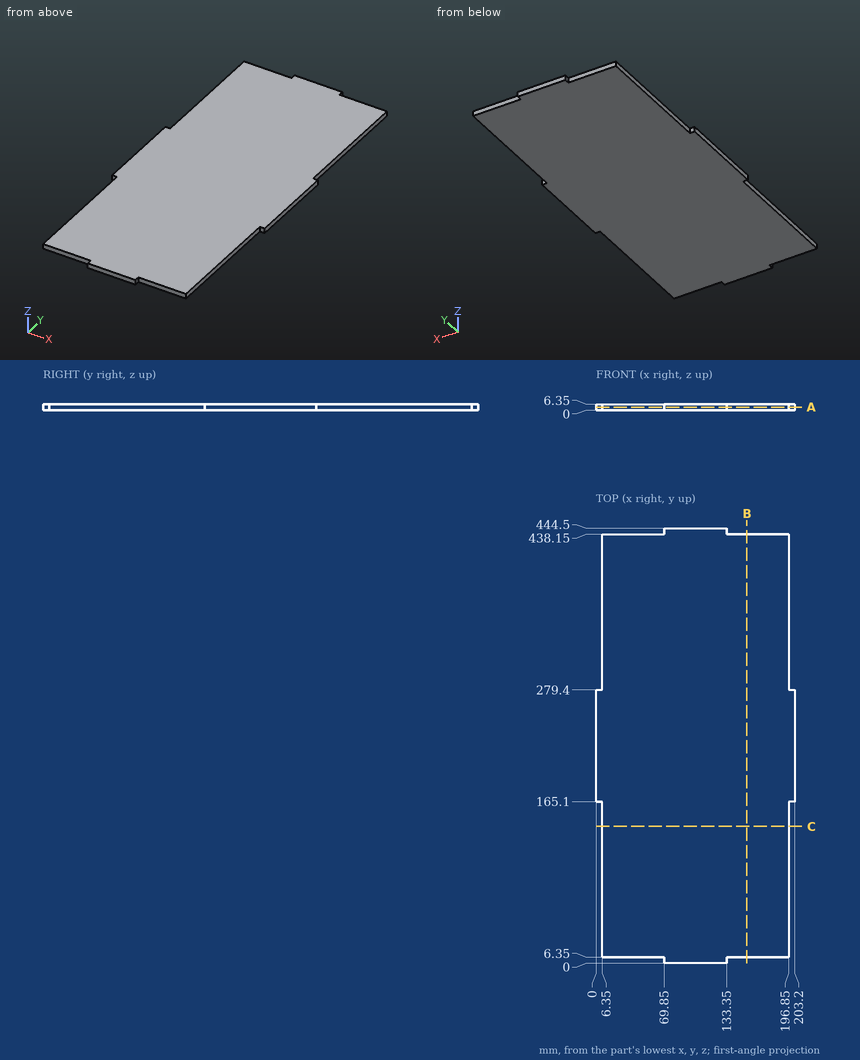
Could you check a few things on this drawing? It's one solid part, dimensions in mm from its lowest x, y, z. Give positions to 0.01 mm unless a question says otherwise; leave off trailing zeros. Order: outer loops, then holes, each group sorted by start corner. A loop starts at its lowest first (then second) coordinate and runs counter-clockwise, first axis right, second up. Notation, with made-up numbers: M -31,71.25 L 3,71.25 A32 cw 3,98.25 Z; hole C -15,-20.5 d11. An arc over 180 degrees is marked long. Use one line per item in the form item = value.
Item 1: If I drill on line 1 along X through (y, z) = (107.5, 0.5); line 2 along Y through (x, z) = (150, 1.75), over which ranges is the centre line in solid material (lowest first)? Write a range as [from, to].
Values follow:
line_1 = [6.35, 196.85]
line_2 = [6.35, 438.15]
Item 2: Will these pins go through, and if not, where does the flat tip stop? pin 1 Ø3 at (y, z) = (440, 2.5) entering from +X; pin 2 Ø1.9 at (x, z) = (174.5, 2.5) entering from +Y; pin 3 Ø3 at (y, z) = (440, 2.5) entering from -X.
Values follow:
pin_1 = 133.35
pin_2 = 438.15
pin_3 = 69.85
Item 3: If we section it at A-A, the plane z = 3.25: Write out the boundary of the cut face in (x, y), and give its area (3 significant figures).
Values follow:
outline = M 0,165.1 L 6.35,165.1 L 6.35,6.35 L 69.85,6.35 L 69.85,0 L 133.35,0 L 133.35,6.35 L 196.85,6.35 L 196.85,165.1 L 203.2,165.1 L 203.2,279.4 L 196.85,279.4 L 196.85,438.15 L 133.35,438.15 L 133.35,444.5 L 69.85,444.5 L 69.85,438.15 L 6.35,438.15 L 6.35,279.4 L 0,279.4 Z
area = 84,500 mm^2
Item 4: If we section it at C-C, the plane y = 140: Write out the boundary of the cut face in (x, z), and give its area (3 significant figures).
Values follow:
outline = M 6.35,0 L 196.85,0 L 196.85,6.35 L 6.35,6.35 Z
area = 1,210 mm^2
Item 5: If we section it at B-B, the plane x = 154: Write out the boundary of the cut face in (y, z).
Values follow:
outline = M 6.35,0 L 438.15,0 L 438.15,6.35 L 6.35,6.35 Z
